from build123d import *

# Parameters (mm, degrees)
SALIENTE_EXTRUIR1_DEPTH = 5
REDONDEO1_R             = 4
CROQUIS2_R              = 1.75
CORTAR_EXTRUIR1_DEPTH   = 99.138932132
REDONDEO2_R             = 1.5
REDONDEO3_R             = 4.5
REDONDEO4_R             = 1.5
REDONDEO5_R             = 1


with BuildPart() as part:
    # Croquis1 → Saliente-Extruir1 (new, symmetric)
    with BuildSketch(Plane.XY):
        Polygon((0, 0), (11, 0), (11, 50.5), (73, 50.5), (73, 0), (84, 0), (84, 3), (76, 3), (76, 53.5), (8, 53.5), (8, 3), (0, 3), align=None)
    extrude(amount=SALIENTE_EXTRUIR1_DEPTH, both=True)

    # Redondeo1
    redondeo1_edges = [part.edges().sort_by_distance(p)[0] for p in [
        (84, 1.5, -5),
        (0, 1.5, -5),
        (84, 1.5, 5),
        (0, 1.5, 5),
    ]]
    fillet(redondeo1_edges, radius=REDONDEO1_R)

    # Croquis2 → Cortar-Extruir1 (cut, through all)
    with BuildSketch(Plane(origin=(0, 3, 0), x_dir=(1, 0, 0), z_dir=(0, 1, 0))):
        with Locations(Location((79.5, 0, 0), (0, 0, 180))):
            Circle(CROQUIS2_R)
    cortar_extruir1 = extrude(amount=-CORTAR_EXTRUIR1_DEPTH, mode=Mode.SUBTRACT)

    # Simetría1: Cortar-Extruir1 across plane
    add(cortar_extruir1.mirror(Plane(origin=(42, 0, 0), x_dir=(0, 0, 1), z_dir=(1, 0, 0))), mode=Mode.SUBTRACT)

    # Redondeo2
    redondeo2_edges = [part.edges().sort_by_distance(p)[0] for p in [
        (73, 50.5, 0),
        (11, 50.5, 0),
    ]]
    fillet(redondeo2_edges, radius=REDONDEO2_R)

    # Redondeo3
    redondeo3_edges = [part.edges().sort_by_distance(p)[0] for p in [
        (8, 53.5, 0),
        (76, 53.5, 0),
    ]]
    fillet(redondeo3_edges, radius=REDONDEO3_R)

    # Redondeo4
    redondeo4_edges = [part.edges().sort_by_distance(p)[0] for p in [
        (73, 0, 0),
        (11, 0, 0),
    ]]
    fillet(redondeo4_edges, radius=REDONDEO4_R)

    # Redondeo5
    redondeo5_edges = [part.edges().sort_by_distance(p)[0] for p in [
        (8, 3, 0),
        (76, 3, 0),
    ]]
    fillet(redondeo5_edges, radius=REDONDEO5_R)


solid = part.part
Can you work these out from the model? Positions are in its coordinate system, mm. A direction names the side the tool comes from. Coordinates: 2 decimals unless noted, no trailing zeros. Order: outer loops, then holes, each group sorted by start corner. A loop starts at its lowest first (then second) coordinate and runs counter-clockwise, first axis right, second up. Notation, with made-up numbers: M 45,77.25 L 103,77.25 A37 cw 103,114.25 Z; hole C 54.5,-22.5 d8. An arc over 180 degrees is marked long. Answer as CSV lines item,"result".
(1) Please list where these lines run through material, in increasing order: L1, parallel to X at y = 43, z = 0.75; L2, parallel to Y at x = 54.5, z = 2; L3, parallel to Z at x = 4, y = 1.
Geometry check:
L1,"8 to 11, 73 to 76"
L2,"50.5 to 53.5"
L3,"-5 to -1.68, 1.68 to 5"
(2) I'm going to push flat-ended pins straight in: pin 1 (2 mm diameter, centred on x = 3, z = 2, fed in from +Y); pin 2 (5.5 mm diameter, centred on x = 79.5, z = 0, fed in from -Y); pin 3 (5 mm diameter, centred on x = 56.5, z = -2, fed in from -Y); pin 4 (5.5 mm diameter, centred on x = 79, z = 2.5, fed in from +Y). Where does each tip first touch, or does it pass through?
Geometry check:
pin 1,"y = 3"
pin 2,"y = 0"
pin 3,"y = 50.5"
pin 4,"y = 3.34"
(3) Suppose I cut it at B-B on z = 0. Please give me the cut outline in (x, y), plus the area to 3 significant figures.
Geometry check:
outline,"M 0,0 L 2.75,0 L 2.75,3 L 0,3 Z; M 6.25,0 L 9.5,0 A1.5 ccw 11,1.5 L 11,49 A1.5 cw 12.5,50.5 L 71.5,50.5 A1.5 cw 73,49 L 73,1.5 A1.5 ccw 74.5,0 L 77.75,0 L 77.75,3 L 77,3 A1 cw 76,4 L 76,49 A4.5 ccw 71.5,53.5 L 12.5,53.5 A4.5 ccw 8,49 L 8,4 A1 cw 7,3 L 6.25,3 Z; M 81.25,0 L 84,0 L 84,3 L 81.25,3 Z"
area,"526 mm^2"
(4) On a 3-axis mill with a long thin cutter (end or side, diameter ignored), from which of +Z, -Z, +X, -X, +Y, -Y can I reach the whole of each face in a straight line? I mean faces 1 (the flat face through (11, 25, 0)), 2 (the flat face through (2.8, 3, -1)), 3 (the cylindrical face through (1.141, 1.479, 3.797)), 4 (the flat face through (81.3, 3, -1)), 5 (the flat face through (77, 0, 0)). Say none if no direction works.
Geometry check:
face 1,"+Z, -Z, -Y"
face 2,"+Z, -Z, -X, +Y"
face 3,"+Z, -X, +Y, -Y"
face 4,"+Z, -Z, +X, +Y"
face 5,"+Z, -Z, +X, -X, -Y"
(5) Suppose I cut it at A-A on y = 10. Please give me the cut outline in (x, z), plus the area to 3 significant figures.
Geometry check:
outline,"M 8,-5 L 11,-5 L 11,5 L 8,5 Z; M 73,-5 L 76,-5 L 76,5 L 73,5 Z"
area,"60.0 mm^2"
(6) If we mould it in two halves opening along X, with no side actions, what happens to faces 6 (the flat face through (36, 51, -5)), 7 (the cylindrical face through (74.647, 52.217, 0.07)), 8 (the flat face through (42, 50.5, 0))? For each: released by +X, released by -X, zero draft, split by the parting line, or undercut.
Geometry check:
face 6,"zero draft"
face 7,"released by +X"
face 8,"undercut"
